Read the model definition and answer for the solid it produces. Units are mm, in the model's axes. A direction names the side the tool comes from. Give positions to 0.01 mm unless a question says otherwise; leave off trailing zeros. Order: outer loops, then holes, each group sorted by start corner. A loop starts at its lowest first (then second) coordinate and runs counter-clockwise, first axis right, second up. Notation, with made-up numbers: (-6.5, 22) - (28.5, 22) arc R21 cw to (28.5, 36) - close; hole circle Ø3 at (-20.75, 52.5). An arc over 180 degrees is marked (long way). Return JSON: item names as keys, results as strings.
```python
from build123d import *

# Parameters (mm, degrees)
F0_R     = 19.5
F1_DEPTH = 3.175


# Not quite as in the source:
# - a length typed as a fraction of an inch, garbled in the dataset ("3 / 203.2 mm" for 3/8 in), is restored


with BuildPart() as f1:
    # F0 (on Front) → F1 (new body)
    with BuildSketch(Plane.XZ):
        Circle(F0_R)
        with BuildLine():
            ThreePointArc((1.5, 14.9248115566), (10.6066017178, 10.6066017178), (14.9248115566, 1.5))
            Line((14.9248115566, 1.5), (17.9248115566, 1.5))
            Line((17.9248115566, 1.5), (17.9248115566, -1.5))
            Line((17.9248115566, -1.5), (14.9248115566, -1.5))
            ThreePointArc((14.9248115566, -1.5), (10.6066017178, -10.6066017178), (1.5, -14.9248115566))
            Line((1.5, -14.9248115566), (1.5, -17.9248115566))
            Line((1.5, -17.9248115566), (-1.5, -17.9248115566))
            Line((-1.5, -17.9248115566), (-1.5, -14.9248115566))
            ThreePointArc((-1.5, -14.9248115566), (-10.6066017178, -10.6066017178), (-14.9248115566, -1.5))
            Line((-14.9248115566, -1.5), (-17.9248115566, -1.5))
            Line((-17.9248115566, -1.5), (-17.9248115566, 1.5))
            Line((-17.9248115566, 1.5), (-14.9248115566, 1.5))
            ThreePointArc((-14.9248115566, 1.5), (-10.6066017178, 10.6066017178), (-1.5, 14.9248115566))
            Line((-1.5, 14.9248115566), (-1.5, 17.9248115566))
            Line((-1.5, 17.9248115566), (1.5, 17.9248115566))
            Line((1.5, 17.9248115566), (1.5, 14.9248115566))
        make_face(mode=Mode.SUBTRACT)
    extrude(amount=F1_DEPTH)


solid = f1.part
```
Q1. A cutting plane is placed at B-B (z = 0). Write down the section's boundary in (x, y) (3 decimals).
Values:
{"outline": "(-19.5, -3.175) - (-17.925, -3.175) - (-17.925, 0) - (-19.5, 0) - close; (17.925, -3.175) - (19.5, -3.175) - (19.5, 0) - (17.925, 0) - close"}
Q2. Given pin 1 (0.9 mm diameter, centred on y = -2, z = 0.5, fed in from +X); pin 2 (1.5 mm diameter, centred on y = -2, z = 8, fed in from +X); pin 3 (0.9 mm diameter, centred on y = -2, z = 16, fed in from +X); pin 4 (0.9 mm diameter, centred on x = 16.5, y = -2.5, fed in from -Z), each flat-ended and moving along its own axis, determine where each tip first touches the part or whether it passes through.
Values:
{"pin 1": "stops at x = 19.5", "pin 2": "stops at x = 18.1", "pin 3": "stops at x = 11.77", "pin 4": "stops at z = -11.07"}
Q3. Consider L1, parallel to X at y = -2.25, z = -5.5; L2, parallel to Z at x = 13, y = -2.65; L3, parallel to X at y = -1.6, z = 11.5. Determine where each line is inside the solid, lowest interval first.
Values:
{"L1": "x = -18.71 to -13.96, 13.96 to 18.71", "L2": "z = -14.53 to -7.48, 7.48 to 14.53", "L3": "x = -15.75 to -9.63, 9.63 to 15.75"}
Q4. For faces 1 (the flat face through (17.925, -2, 0)), 2 (the flat face through (11.5, 0, -10)), determine the directions among +Z, -Z, +X, -X, +Y, -Y from which every point of the face is accessible in a straight line to the end or side of a thin tool.
Values:
{"face 1": "+Y, -Y", "face 2": "+Z, -Z, +X, -X, +Y"}
Q5. A cutting plane is placed at A-A (x = 0). Write down the section's boundary in (y, z) (3 decimals), and give its area (3 significant figures).
Values:
{"outline": "(-3.175, -19.5) - (0, -19.5) - (0, -17.925) - (-3.175, -17.925) - close; (-3.175, 17.925) - (0, 17.925) - (0, 19.5) - (-3.175, 19.5) - close", "area": "10.0 mm²"}
Q6. Determine the mould class of faces 3 (the flat face through (11.5, -3.175, -10)), 4 (the flat face through (-17.925, -2, 0)), 5 (the cylindrical face through (-2.539, -1.565, 19.334)) for opening direction X: released by +X, released by -X, zero draft, split by the parting line, or undercut.
Values:
{"face 3": "zero draft", "face 4": "undercut", "face 5": "split by the parting line"}
Q7. A cutting plane is placed at C-C (y = -0.65). Write down the section's boundary in (x, z), and give its area (3 significant figures).
Values:
{"outline": "circle Ø39 at (0, 0); hole (-17.92, -1.5) - (-14.92, -1.5) arc R15 ccw to (-1.5, -14.92) - (-1.5, -17.92) - (1.5, -17.92) - (1.5, -14.92) arc R15 ccw to (14.92, -1.5) - (17.92, -1.5) - (17.92, 1.5) - (14.92, 1.5) arc R15 ccw to (1.5, 14.92) - (1.5, 17.92) - (-1.5, 17.92) - (-1.5, 14.92) arc R15 ccw to (-14.92, 1.5) - (-17.92, 1.5) - close", "area": "452 mm²"}
